```python
from build123d import *

# Parameters (mm, degrees)
F0_R     = 18.5
F0_R_2   = 10
F1_DEPTH = 9
F2_R     = 16.5
F2_R_2   = 12.5
F3_DEPTH = 0.5
F4_R     = 16.5
F4_R_2   = 12.5
F5_DEPTH = 0.5


with BuildPart() as f1:
    # F0 (on Front) → F1 (new body)
    with BuildSketch(Plane.XZ):
        Circle(F0_R)
        Circle(F0_R_2, mode=Mode.SUBTRACT)
    extrude(amount=F1_DEPTH)

    # F2 (on face) → F3 (cut)
    with BuildSketch(Plane.XZ.offset(9)):
        Circle(F2_R)
        Circle(F2_R_2, mode=Mode.SUBTRACT)
    extrude(amount=-F3_DEPTH, mode=Mode.SUBTRACT)

    # F4 (on Front) → F5 (cut)
    with BuildSketch(Plane.XZ):
        Circle(F4_R)
        Circle(F4_R_2, mode=Mode.SUBTRACT)
    extrude(amount=F5_DEPTH, mode=Mode.SUBTRACT)


solid = f1.part
```
The listing builds one solid part. Answer for the finished solid, in the listing's coordinates (mm). A direction names the side the tool comes from. Coordinates: 2 decimals unless noted, no trailing zeros. Write each loop counter-clockwise with the first axis right and the second up, starting at its lowest first coordinate (ties: lowest second). Pieces come first, ordered by that corner, then holes. Notation, with made-up numbers: (53.5, 62.5) - (103.5, 62.5) arc R25 cw to (103.5, 100.5) - close; hole circle Ø6 at (86.5, 17.5). An arc over 180 degrees is marked (long way). Return JSON: item names as keys, results as strings. Group by question number.
Q1. The part is cut by section D-D on y = -6.5. Write down the section's boundary in (x, z), and give its area (3 significant figures).
Q2. The part is cut by section A-A on z = 0. Write down the section's boundary in (x, y).
Q3. Which of the six approach directions +Z, -Z, +X, -X, +Y, -Y give full straight-line access (tool end or side, diameter ignored) to faces 1 (the cylindrical face through (15.24, -8.75, -6.32)), 2 (the flat face through (-12.3, -0.5, 3.7)), 3 (the flat face through (-0.1, 0, 10.2))?
Q4. The part is cut by section B-B on x = 0. Write down the section's boundary in (y, z), and give its area (3 significant figures).
Q5. For a pull along X with two mould halves and no side action, classify faces 4 (the flat face through (-17, 0, 0)), 5 (the cylindrical face through (11.923, -8.754, 3.755)), 6 (the cylindrical face through (-4.01, -4.44, -18.06)), 7 (the flat face through (-12.3, -8.5, 3.7)) as +X half, -X half, draft (parallel to the pull), parting line (faces both ways), or undercut.
Q6. Find the intervals of material crossed by line 1 along Z through (x, y) = (0, -3); line 2 along Y through (x, z) = (2, 12.5); line 3 along X through (y, z) = (-8, 6), in increasing order. Write a range as [from, to].
Q7. Flat-ended cylindrical pins translate along their axes: pin 1 Ø16.5 at (x, z) = (7.5, 0) entering from -Y; pin 2 Ø1 at (x, y) = (11.5, -2) entering from +Z; pin 3 Ø3 at (x, z) = (-0.5, -8) entering from +Y; pin 4 Ø3 at (y, z) = (-6, -11) entering from -X. Find the tip coordinate at first contact, or state that the pin passes through.
Q8. The part is cut by section C-C on z = -11. Write down the section's boundary in (x, y), and give its area (3 significant figures).
Evaluation:
{
 "1": {"outline": "circle Ø37 at (0, 0); hole circle Ø20 at (0, 0)", "area": "761 mm2"},
 "2": {"outline": "(-18.5, -9) - (-16.5, -9) - (-16.5, -8.5) - (-12.5, -8.5) - (-12.5, -9) - (-10, -9) - (-10, 0) - (-12.5, 0) - (-12.5, -0.5) - (-16.5, -0.5) - (-16.5, 0) - (-18.5, 0) - close; (10, -9) - (12.5, -9) - (12.5, -8.5) - (16.5, -8.5) - (16.5, -9) - (18.5, -9) - (18.5, 0) - (16.5, 0) - (16.5, -0.5) - (12.5, -0.5) - (12.5, 0) - (10, 0) - close"},
 "3": {"face 1": "-Y", "face 2": "+Y", "face 3": "+Z, -Z, +X, -X, +Y"},
 "4": {"outline": "(-9, -18.5) - (0, -18.5) - (0, -16.5) - (-0.5, -16.5) - (-0.5, -12.5) - (0, -12.5) - (0, -10) - (-9, -10) - (-9, -12.5) - (-8.5, -12.5) - (-8.5, -16.5) - (-9, -16.5) - close; (-9, 10) - (0, 10) - (0, 12.5) - (-0.5, 12.5) - (-0.5, 16.5) - (0, 16.5) - (0, 18.5) - (-9, 18.5) - (-9, 16.5) - (-8.5, 16.5) - (-8.5, 12.5) - (-9, 12.5) - close", "area": "145 mm2"},
 "5": {"face 4": "draft", "face 5": "undercut", "face 6": "parting line", "face 7": "undercut"},
 "6": {"line 1": "z = [-18.5, -10], [10, 18.5]", "line 2": "y = [-8.5, -0.5]", "line 3": "x = [-17.5, -8], [8, 17.5]"},
 "7": {"pin 1": "stops at y = -9", "pin 2": "stops at z = 14.87", "pin 3": "passes through", "pin 4": "stops at x = -15.87"},
 "8": {"outline": "(-14.87, -9) - (-12.3, -9) - (-12.3, -8.5) - (-5.94, -8.5) - (-5.94, -9) - (5.94, -9) - (5.94, -8.5) - (12.3, -8.5) - (12.3, -9) - (14.87, -9) - (14.87, 0) - (12.3, 0) - (12.3, -0.5) - (5.94, -0.5) - (5.94, 0) - (-5.94, 0) - (-5.94, -0.5) - (-12.3, -0.5) - (-12.3, 0) - (-14.87, 0) - close", "area": "255 mm2"}
}
